```python
from build123d import *

# Parameters (mm, degrees)
BOSS_EXTRUDE1_DEPTH         = 25.4
F_1_2_CLEARANCE_HOLE1_D     = 13.09624
F_1_2_CLEARANCE_HOLE1_DEPTH = 76.2
F_1_2_CLEARANCE_HOLE1_TIP   = 3.934507437


with BuildPart() as part:
    # Sketch1 → Boss-Extrude1 (new body)
    with BuildSketch(Plane.XY):
        Polygon((0, 0), (-355.6, 0), (-355.6, 6.35), (-292.1, 6.35), (-292.1, 160.451477372), (-230.75738686, 266.7), (-124.84261314, 266.7), (-63.5, 160.451477372), (-63.5, 6.35), (0, 6.35), align=None)
        Polygon((-285.75, 158.75), (-285.75, 6.35), (-69.85, 6.35), (-69.85, 158.75), (-128.50878735, 260.35), (-227.09121265, 260.35), align=None, mode=Mode.SUBTRACT)
    extrude(amount=BOSS_EXTRUDE1_DEPTH)

    # 1/2 Clearance Hole1
    with Locations(Plane(origin=(0, 0, 0), x_dir=(-1, 0, 0), z_dir=(0, -1, 0))):
        with Locations((25.4, -12.7), (330.2, -12.7)):
            Hole(F_1_2_CLEARANCE_HOLE1_D / 2, depth=F_1_2_CLEARANCE_HOLE1_DEPTH)
            with Locations((0, 0, -(F_1_2_CLEARANCE_HOLE1_DEPTH + F_1_2_CLEARANCE_HOLE1_TIP / 2))):  # 118° drill point
                Cone(0, F_1_2_CLEARANCE_HOLE1_D / 2, F_1_2_CLEARANCE_HOLE1_TIP, mode=Mode.SUBTRACT)


solid = part.part
```
The model under review builds one solid part; all positions refer to its coordinate system, in mm. A direction names the side the tool comes from. Round coordinates to 2 decimals unless told otherwise and drop trailing zeros. Loops run counter-clockwise (first coordinate to the right, second up) from the corner with the lowest first, then second, coordinate; pieces in that order, holes last. Notation, with made-up numbers: (-29, 57) - (4, 57) arc R29 ccw to (4, 80) - close; hole circle Ø10 at (20.5, -12.5). An arc over 180 degrees is marked (long way). Write each question's results on one line, items separated by ' | '. Start each with the question number.
Q1. Wall thickness on line 1 along Y through (x, z) = (-221, 9.5); line 2 along X through (y, z) = (15.5, 1.25); line 3 along Z through (x, y) = (-330.2, 2.5): over which ranges is each line inside the solid? List them lowest first. Write a range as [from, to].
Q2. Take a section at B-B on z = 12.7. Give the boundary of the cut face in (x, y).
Q3. Draft analysis for pull direction Y (two halves, no side actions). For faces 1 (the flat face through (-175, 0, 13)), 2 (the flat face through (-94.6, 214.32, 12.52)), 3 (the flat face through (-179, 6.35, 13)), state which applies: pulls with the +Y half, pulls with the -Y half, needs draft (parallel to the pull), parting line crosses it, or undercut.
Q4. Take a section at C-C on y = 56.5. Give the boundary of the cut face in (x, z).
Q5. Take a section at A-A on x = -25.4. Give the boundary of the cut face in (y, z).
Q6. Tool access review of faces 4 (the cylindrical face through (-336.74, 3.22, 12.41)), 5 (the flat face through (-292.1, 82, 13)), 6 (the flat face through (-63.5, 84, 13)), 7 (the flat face through (-256.01, 210.26, 12.52)): name each direction out of +Z, -Z, +X, -X, +Y, -Y from which nothing blocks a thin tool from reaching the whole face with its end or side.
Q7. Insertion check: P1, Ø15, axis at x = -330.2, z = 12.7, coming from the +Y side; P2, Ø10, axis at y = 82.5, z = 13.5, coming from the +X side; P3, Ø12.5, axis at y = 109, z = 14, coming from the -X side. Each pin has a flat end and moves straight along its axis. Give the tip position at first contact, or say it passes through.
Data:
1) line 1: y = [0, 6.35], [260.35, 266.7] | line 2: x = [-292.1, -285.75], [-69.85, -63.5] | line 3: z = [0, 6.15], [19.25, 25.4]
2) outline: (-355.6, 0) - (-336.75, 0) - (-336.75, 6.35) - (-355.6, 6.35) - close; (-323.65, 0) - (-31.95, 0) - (-31.95, 6.35) - (-63.5, 6.35) - (-63.5, 160.45) - (-124.84, 266.7) - (-230.76, 266.7) - (-292.1, 160.45) - (-292.1, 6.35) - (-323.65, 6.35) - close; (-18.85, 0) - (0, 0) - (0, 6.35) - (-18.85, 6.35) - close; hole (-285.75, 6.35) - (-69.85, 6.35) - (-69.85, 158.75) - (-128.51, 260.35) - (-227.09, 260.35) - (-285.75, 158.75) - close
3) face 1: pulls with the -Y half | face 2: pulls with the +Y half | face 3: undercut
4) outline: (-292.1, 0) - (-285.75, 0) - (-285.75, 25.4) - (-292.1, 25.4) - close; (-69.85, 0) - (-63.5, 0) - (-63.5, 25.4) - (-69.85, 25.4) - close
5) outline: (0, 0) - (6.35, 0) - (6.35, 6.15) - (0, 6.15) - close; (0, 19.25) - (6.35, 19.25) - (6.35, 25.4) - (0, 25.4) - close
6) face 4: +Y, -Y | face 5: +Z, -Z, -X, +Y | face 6: +Z, -Z, +X, +Y | face 7: +Z, -Z
7) P1: stops at y = 6.35 | P2: stops at x = -63.5 | P3: stops at x = -292.1
